```python
from build123d import *

# Parameters (mm, degrees)
F1_DEPTH  = 2000
F3_DEPTH  = 600.001
F6_DEPTH  = 1995.001
F8_DEPTH  = 1410
F10_DEPTH = 800
F12_DEPTH = 1995.001


with BuildPart() as f1:
    # F0 (on Front) → F1 (new body)
    with BuildSketch(Plane.XZ):
        with BuildLine():
            ThreePointArc((1355.2, 2268.467492), (1322.870911, 2382.422107), (1235.516548, 2462.422356))
            ThreePointArc((1235.516548, 2462.422356), (634.843055, 2680.85794), (0, 2755))
            ThreePointArc((0, 2755), (-634.843055, 2680.85794), (-1235.516548, 2462.422356))
            ThreePointArc((-1235.516548, 2462.422356), (-1322.870911, 2382.422107), (-1355.2, 2268.467492))
            Line((-1355.2, 2268.467492), (-1357.791007, 2155))
            Line((-1357.791007, 2155), (0, 2155))
            Line((0, 2155), (1357.791007, 2155))
            Line((1357.791007, 2155), (1355.2, 2268.467492))
        make_face()
    extrude(amount=-F1_DEPTH)

    # F2 (on face) → F3 (cut, through all)
    with BuildSketch(Plane(origin=(0, 0, 2155), x_dir=(1, 0, 0), z_dir=(0, 0, -1))):
        with BuildLine():
            ThreePointArc((-1357.791007, -50), (0, -5), (1357.791007, -50))
            Line((1357.791007, -50), (1357.791007, 0))
            Line((1357.791007, 0), (-1357.791007, 0))
            Line((-1357.791007, 0), (-1357.791007, -50))
        make_face()
    extrude(amount=-F3_DEPTH, mode=Mode.SUBTRACT)

    # F5 (on face) → F6 (cut, through all)
    with BuildSketch(Plane(origin=(0, 2000, 0), x_dir=(-1, 0, 0), z_dir=(0, 1, 0))):
        with BuildLine():
            Line((-439.645053, 2719.694326), (0, 2719.694326))
            Line((0, 2719.694326), (439.645053, 2719.694326))
            ThreePointArc((439.645053, 2719.694326), (220.530193, 2746.159397), (0, 2755))
            ThreePointArc((0, 2755), (-220.530193, 2746.159397), (-439.645053, 2719.694326))
        make_face()
    extrude(amount=-F6_DEPTH, mode=Mode.SUBTRACT)

    # F7 (on face) → F8 (join)
    with BuildSketch(Plane(origin=(0, 2000, 0), x_dir=(-1, 0, 0), z_dir=(0, 1, 0))):
        with BuildLine():
            ThreePointArc((-93.5, 2753.412928), (0, 2755), (93.5, 2753.412928))
            Line((93.5, 2753.412928), (93.5, 2791.694326))
            Line((93.5, 2791.694326), (83.107695, 2809.694326))
            Line((83.107695, 2809.694326), (0, 2809.694326))
            Line((0, 2809.694326), (-83.107695, 2809.694326))
            Line((-83.107695, 2809.694326), (-93.5, 2791.694326))
            Line((-93.5, 2791.694326), (-93.5, 2753.412928))
        make_face()
        with BuildLine():
            Line((-93.5, 2719.694326), (93.5, 2719.694326))
            Line((93.5, 2719.694326), (93.5, 2753.412928))
            ThreePointArc((93.5, 2753.412928), (0, 2755), (-93.5, 2753.412928))
            Line((-93.5, 2753.412928), (-93.5, 2719.694326))
        make_face()
    extrude(amount=-F8_DEPTH)

    # F9 (on face) → F10 (cut)
    with BuildSketch(Plane(origin=(0, 2000, 0), x_dir=(-1, 0, 0), z_dir=(0, 1, 0))):
        with BuildLine():
            ThreePointArc((1355.2, 2268.467492), (1322.870911, 2382.422107), (1235.516548, 2462.422356))
            ThreePointArc((1235.516548, 2462.422356), (847.401212, 2621.437809), (439.645053, 2719.694326))
            Line((439.645053, 2719.694326), (93.5, 2719.694326))
            Line((93.5, 2719.694326), (93.5, 2791.694326))
            Line((93.5, 2791.694326), (83.107695, 2809.694326))
            Line((83.107695, 2809.694326), (-83.107695, 2809.694326))
            Line((-83.107695, 2809.694326), (-93.5, 2791.694326))
            Line((-93.5, 2791.694326), (-93.5, 2719.694326))
            Line((-93.5, 2719.694326), (-439.645053, 2719.694326))
            ThreePointArc((-439.645053, 2719.694326), (-847.401212, 2621.437809), (-1235.516548, 2462.422356))
            ThreePointArc((-1235.516548, 2462.422356), (-1322.870911, 2382.422107), (-1355.2, 2268.467492))
            Line((-1355.2, 2268.467492), (-1357.791007, 2155))
            Line((-1357.791007, 2155), (1357.791007, 2155))
            Line((1357.791007, 2155), (1355.2, 2268.467492))
        make_face()
    extrude(amount=-F10_DEPTH, mode=Mode.SUBTRACT)

    # F11 (on face) → F12 (cut, through all)
    with BuildSketch(Plane(origin=(0, 2000, 0), x_dir=(-1, 0, 0), z_dir=(0, 1, 0))):
        with BuildLine():
            Line((735.527022, 2655), (-735.527022, 2655))
            ThreePointArc((-735.527022, 2655), (-990.214485, 2570.894839), (-1235.516548, 2462.422356))
            ThreePointArc((-1235.516548, 2462.422356), (-1322.870911, 2382.422107), (-1355.2, 2268.467492))
            Line((-1355.2, 2268.467492), (-1357.791007, 2155))
            Line((-1357.791007, 2155), (1357.791007, 2155))
            Line((1357.791007, 2155), (1355.2, 2268.467492))
            ThreePointArc((1355.2, 2268.467492), (1322.870911, 2382.422107), (1235.516548, 2462.422356))
            ThreePointArc((1235.516548, 2462.422356), (990.214485, 2570.894839), (735.527022, 2655))
        make_face()
    extrude(amount=-F12_DEPTH, mode=Mode.SUBTRACT)


solid = f1.part
```
Check sheet for the modelled part. Datum: model origin and axes. Units: mm. A direction names the side the tool comes from. Round coordinates to 2 decimals unless told otherwise and drop trailing zeros. Loops run counter-clockwise (first coordinate to the right, second up) from the corner with the lowest first, then second, coordinate; pieces in that order, holes last. Notation, with made-up numbers: (22.5, 26) - (68.5, 26) arc R32 cw to (68.5, 65) - close; hole circle Ø4 at (-2.5, -29). An arc over 180 degrees is marked (long way). Write item = value, one per line. Start each with the question number.
Q1. Section check D-D (x = -45). Record the boundary of the cut face in (y, z).
Q2. Thickness scan on L1, parallel to X at y = 801, z = 2724.5; L2, parallel to Z at x = -293.5, y = 289.5; L3, parallel to Y at x = -45, z = 2756. Record the ranges inside material, lowest first.
Q3. Section check C-C (z = 2697.5). Record the boundary of the cut face in (x, y), plus the area to 3 significant figures.
Q4. Access from +Z, -Z, +X, -X, +Y, -Y to the whole of each face (thin tool, end or side, straight path). Record for faces 1 (the face through (-93.5, 899, 2755)), 2 (the face through (1, 590, 2765)), 3 (the face through (93.5, 899, 2756)).
Q5. Section check A-A (y = 700). Record the boundary of the cut face in (x, z).
Derived:
q1.outline = (5.05, 2655) - (1200, 2655) - (1200, 2809.69) - (590, 2809.69) - (590, 2719.69) - (5.05, 2719.69) - close
q2.L1 = -93.5 to 93.5
q2.L2 = 2655 to 2719.69
q2.L3 = 590 to 1200
q3.outline = (-559.93, 12.65) arc R20506.9 ccw to (559.93, 12.65) - (559.93, 1200) - (-559.93, 1200) - close
q3.area = 1,340,000 mm^2
q4.face_1 = +Z, -X, +Y, -Y
q4.face_2 = +Z, +X, -X, -Y
q4.face_3 = +Z, +X, +Y, -Y
q5.outline = (-735.53, 2655) - (735.53, 2655) arc R2755 ccw to (439.65, 2719.69) - (93.5, 2719.69) - (93.5, 2791.69) - (83.11, 2809.69) - (-83.11, 2809.69) - (-93.5, 2791.69) - (-93.5, 2719.69) - (-439.65, 2719.69) arc R2755 ccw to start
